CAD build for the part. Positions are in the model's coordinates, mm. A direction names the side the tool comes from. Give positions to 0.01 mm unless a question says otherwise; leave off trailing zeros. Order: outer loops, then holes, each group sorted by start corner. A loop starts at its lowest first (then second) coordinate and runs counter-clockwise, first axis right, second up. Notation, with made-up numbers: M 37.25,38.25 L 84.25,38.25 A21 ccw 84.25,64.25 Z; hole C 36.5,-26 d9. An arc over 180 degrees is marked long. Put each result on its own line as item: value. Start each with the question number.
1) Cut at C-C (z = -17). Write the cut outline in (x, y), and give its area (3 significant figures).
2) Pin check, flat tips, straight feed: pin 1 (6 mm diameter, centred on x = 1, y = -1.5, fed in from -Z); pin 2 (4 mm diameter, centred on x = 9.5, y = -4.5, fed in from -Z); pin 3 (12 mm diameter, centred on x = 1.5, z = -22.5, fed in from -Y); pin 4 (1.2 mm diameter, centred on y = 0, z = -10, fed in from +X). Stop position of each tip, or through.
3) Two-plate mould, pull along Z, no slides. Class faces 4 (the face through (0, -1, 0)), 5 (the face through (0, -4, 1.25)), 6 (the face through (2, 4, -13.25)): released by +Z, released by -Z, zero draft, split by the parting line, or undercut.
4) Cut at D-D (x = -8.5). Write the cut outline in (y, z), and give its area (3 significant figures).
5) Tool access for faces 1 (the face through (2.192, 4.214, -8.264)), 2 (the face through (0, -8, -1.25)), 3 (the face through (-2.5, 0.1, -26.25)): list every direction of +Z, -Z, +X, -X, +Y, -Y with a clear straight run to the whole face (end or side of a thin tool).
6) Drill centre lines: line 1 (Y direction, x = 0, z = 0.15); line 2 (Z direction, x = -3.5, y = 3); line 3 (Z direction, x = 0.5, y = -12). Where is each one in solid material? Low to high. Write a range as [from, to].
7) Cut at A-A (z = -8). Write the cut outline in (x, y), and give its area (3 significant figures).
8) Cut at B-B (y = 8). Write the cut outline in (x, z).
```python
from build123d import *

# Parameters (mm, degrees)
CROQUIS2_R              = 17.5
SALIENTE_EXTRUIR1_DEPTH = 1.25
SALIENTE_EXTRUIR2_DEPTH = 25
CROQUIS4_R              = 1
CORTAR_EXTRUIR1_DEPTH   = 15
CROQUIS7_R              = 1.5
CORTAR_EXTRUIR2_DEPTH   = 10
CROQUIS8_W              = 1.5
CROQUIS8_H              = 2
CROQUIS8_W_2            = 1


with BuildPart() as part:
    # Croquis2 → Saliente-Extruir1 (new, symmetric)
    with BuildSketch(Plane.XY):
        Circle(CROQUIS2_R)
    extrude(amount=SALIENTE_EXTRUIR1_DEPTH, both=True)

    # Croquis3 → Saliente-Extruir2 (add)
    with BuildSketch(Plane(origin=(0, 0, -1.25), x_dir=(-1, 0, 0), z_dir=(0, 0, -1))):
        with BuildLine():
            ThreePointArc((5.75, 0), (4.065863992, 4.065863992), (0, 5.75))
            Line((0, 5.75), (0, 2.75))
            ThreePointArc((0, 2.75), (1.055947953, 2.53918765), (1.95, 1.939071943))
            ThreePointArc((1.95, 1.939071943), (2.542144764, 1.048808848), (2.75, 0))
            ThreePointArc((2.75, 0), (2.542144764, -1.048808848), (1.95, -1.939071943))
            ThreePointArc((1.95, -1.939071943), (1.055947953, -2.53918765), (0, -2.75))
            Line((0, -2.75), (0, -5.75))
            ThreePointArc((0, -5.75), (4.065863992, -4.065863992), (5.75, 0))
        make_face()
        with BuildLine():
            Line((0, 2.75), (0, 5.75))
            ThreePointArc((0, 5.75), (-5.75, 0), (0, -5.75))
            Line((0, -5.75), (0, -2.75))
            ThreePointArc((0, -2.75), (-1.055947953, -2.53918765), (-1.95, -1.939071943))
            ThreePointArc((-1.95, -1.939071943), (-2.75, 0), (-1.95, 1.939071943))
            ThreePointArc((-1.95, 1.939071943), (-1.055947953, 2.53918765), (0, 2.75))
        make_face()
        with BuildLine():
            Line((-1.95, -1.939071943), (-1.95, 1.939071943))
            ThreePointArc((-1.95, 1.939071943), (-2.75, 0), (-1.95, -1.939071943))
        make_face()
        with BuildLine():
            ThreePointArc((2.75, 0), (2.542144764, 1.048808848), (1.95, 1.939071943))
            Line((1.95, 1.939071943), (1.95, -1.939071943))
            ThreePointArc((1.95, -1.939071943), (2.542144764, -1.048808848), (2.75, 0))
        make_face()
    extrude(amount=SALIENTE_EXTRUIR2_DEPTH)

    # Croquis4 → Cortar-Extruir1 (cut)
    with BuildSketch(Plane.XY.offset(1.25)):
        Circle(CROQUIS4_R)
    extrude(amount=-CORTAR_EXTRUIR1_DEPTH, mode=Mode.SUBTRACT)

    # Croquis7 → Cortar-Extruir2 (cut)
    with BuildSketch(Plane.XY.offset(1.25)):
        with Locations((0, 8)):
            Circle(CROQUIS7_R)
    extrude(amount=-CORTAR_EXTRUIR2_DEPTH, mode=Mode.SUBTRACT)

    # Croquis8 → Cortar-Revolución1 (revolve, cut)
    with BuildSketch(Plane(origin=(0, 0, 0), x_dir=(1, 0, 0), z_dir=(0, 1, 0))):
        with Locations((5, 14.25)):
            Rectangle(CROQUIS8_W, CROQUIS8_H)
        with Locations((5.25, 8.25)):
            Rectangle(CROQUIS8_W_2, CROQUIS8_H)
    revolve(axis=Axis((0, 0, 0), (0, 0, -1)), mode=Mode.SUBTRACT)


solid = part.part
```
Solution:
1. outline: C 0,0 d11.5; hole M -1.95,-1.94 A2.75 ccw 1.95,-1.94 L 1.95,1.94 A2.75 ccw -1.95,1.94 Z
1. area: 84.4 mm²
2. pin 1: z = -26.25
2. pin 2: z = -1.25
2. pin 3: y = -5.75
2. pin 4: x = 5.75
3. face 4: zero draft
3. face 5: released by +Z
3. face 6: undercut
4. outline: M -15.3,-1.25 L 15.3,-1.25 L 15.3,1.25 L -15.3,1.25 Z
4. area: 76.5 mm²
5. face 1: none
5. face 2: -Z
5. face 3: -Z, +X, -X, +Y, -Y
6. line 1: [-17.5, -1], [1, 6.5], [9.5, 17.5]
6. line 2: [-26.25, -15.25], [-13.25, 1.25]
6. line 3: [-1.25, 1.25]
7. outline: C 0,0 d9.5; hole M -1.95,-1.94 A2.75 ccw 1.95,-1.94 L 1.95,1.94 A2.75 ccw -1.95,1.94 Z
7. area: 51.4 mm²
8. outline: M -15.56,-1.25 L -1.5,-1.25 L -1.5,1.25 L -15.56,1.25 Z; M 1.5,-1.25 L 15.56,-1.25 L 15.56,1.25 L 1.5,1.25 Z
